from build123d import *

# Parameters (mm, degrees)
F1_DEPTH = 5.8


with BuildPart() as f1:
    # F0 (on Top) → F1 (new body)
    with BuildSketch(Plane.XY):
        Polygon((19.870715, 20.171389), (11.003364, 25.828145), (9.710712, 25.935493), (8.638659, 25.674237), (7.548944, 24.40875), (7.098501, 22.336712), (7.098501, 20.264676), (7.745507, 18.576713), (8.39527, 18.462049), (9.515883, 19.793121), (10.092715, 21.398216), (11.178206, 21.398216), (11.178206, 15.477047), (11.710122, 14.888561), (12.432186, 15.31403), (14.361553, 18.82783), (14.710026, 18.82783), (14.968658, 17.630091), (15.437118, 16.368851), (16.193863, 15.467965), (16.986642, 14.999504), (15.95501, 4.724317), (15.226499, 4.017233), (14.733682, 3.160161), (14.540842, 1.960261), (14.733682, 0.846068), (15.183645, 0), (15.805023, -0.675234), (14.859016, -12.881954), (14.056012, -13.806167), (13.617913, -16.297314), (12.787792, -16.297314), (10.52028, -10.248602), (9.737968, -9.775993), (8.959359, -10.581703), (8.959359, -18.013308), (7.532651, -18.013308), (7.532651, -16.239962), (6.00086, -14.336004), (5.722645, -14.336004), (4.844186, -15.200062), (4.586618, -16.215181), (4.586618, -17.39696), (5.071451, -18.609043), (5.722946, -19.396897), (7.289982, -20.181168), (23.513971, -20.668361), (25.093786, -20.388072), (26.864707, -19.636385), (28.431782, -18.527966), (30.902525, -17.158909), (31.791739, -17.158909), (32.466684, -16.912501), (33.098772, -16.408972), (33.633251, -15.701212), (33.868946, -14.790573), (33.868946, -13.933501), (33.579685, -13.301411), (32.847531, -12.387843), (32.847531, -11.59999), (32.847531, -10.190943), (32.286942, -8.706142), (31.696055, -7.554664), (30.464781, -5.741373), (29.919345, -4.332328), (29.782984, -2.574808), (29.979948, -1.13546), (30.373875, 0.137226), (30.752651, 1.07659), (31.948227, 2.286357), (32.443713, 2.286357), (33.434689, 2.133206), (34.362599, 2.331401), (35.272494, 2.7368), (35.912123, 3.295349), (36.371578, 3.889933), (36.58779, 3.889933), (37.781443, 3.788194), (38.622316, 3.788194), (39.412223, 3.915599), (40.253092, 4.399735), (40.597085, 5.329788), (40.597085, 6.196138), (40.342275, 6.833161), (39.743476, 7.189893), (37.296191, 7.57748), (35.560623, 7.57748), (33.782199, 7.298932), (31.425729, 6.457172), (29.820433, 5.234089), (27.787192, 2.836954), (26.976394, 1.287431), (26.000202, -1.772101), (26.000202, -3.229123), (26.407311, -5.307521), (27.071541, -7.150225), (28.203402, -9.181112), (28.991256, -10.256835), (29.204722, -11.574975), (29.204722, -13.16472), (28.326225, -14.503894), (27.008476, -15.650228), (25.722869, -16.346598), (24.370953, -16.518012), (22.442544, -16.26089), (20.706974, -15.53238), (19.292805, -14.718162), (21.281268, 16.815733), (21.37769, 17.769225), (21.056287, 18.615583), (20.606324, 19.451229), align=None)
    extrude(amount=F1_DEPTH)


solid = f1.part
Design review of the part built by this model. Coordinates are the model's own, in mm. A direction names the side the tool comes from. Round coordinates to 2 decimals unless told otherwise and drop trailing zeros. Write each loop counter-clockwise with the first axis right and the second up, starting at its lowest first coordinate (ties: lowest second). Pieces come first, ordered by that corner, then holes. Notation, with made-up numbers: (49, 46) - (56, 46) arc R29 cw to (56, 84) - close; hole circle Ø3 at (29, -18.5). An arc over 180 degrees is marked (long way). Return JSON: item names as keys, results as strings. Group by question number.
Item 1: The part is to be moulded in two halves that separate along Y. For faces 1 (the face through (34.68, 7.44, 2.86)), 2 (the face through (32.57, -9.46, 2.86)), 3 (the face through (29.65, -17.853, 2.859)), say which applies: pulls with the +Y half, pulls with the -Y half, needs draft (parallel to the pull), parting line crosses it, or undercut.
Item 2: Insertion check: P1, Ø0.7, axis at y = -11.5, z = 4, coming from the +X side; P2, Ø2, axis at x = 27, z = 5, coming from the +Y side; P3, Ø3, axis at x = 20.5, y = 3.5, coming from the +Z side; P4, Ø1.1, axis at x = 8.5, z = 2, coming from the +Y side. Each pin has a flat end and moves straight along its axis. Give the tip position at first contact, or say it passes through.
Item 3: For probe 1 along Y at (x, z) = (23.5, 1); probe 2 along X at (y, z) = (17, 3.05); probe 3 along Y at (x, z) = (33, 0.25), list the stretches that pass through material, from the lowest coordinate up. Write a range as [from, to].
Item 4: We need section B-B on y = 11.5. Write out the cut boundary in (x, z).
Item 5: We need section A-A on x = 18.5. Write out the cut boundary in (y, z).
Item 6: Machinability: for faces 4 (the face through (15.2, 17.01, 2.86)), 5 (the face through (7.099, 21, 3)), 6 (the face through (29.88, -1.87, 2.86)), which of the approach directions +Z, -Z, +X, -X, +Y, -Y give a long, thin tool a straight path to every point of the face, cutting with its end or side? Answer none if there is none.
Model answer:
{
 "1": {"face 1": "pulls with the +Y half", "face 2": "undercut", "face 3": "pulls with the -Y half"},
 "2": {"P1": "stops at x = 32.85", "P2": "stops at y = 3.09", "P3": "stops at z = 5.8", "P4": "stops at y = 25.77"},
 "3": {"probe 1": "y = [-20.67, -16.4]", "probe 2": "x = [11.18, 13.36], [15.2, 21.3]", "probe 3": "y = [-16.49, -12.58], [2.2, 7.02]"},
 "4": {"outline": "(16.64, 0) - (20.95, 0) - (20.95, 5.8) - (16.64, 5.8) - close"},
 "5": {"outline": "(-20.52, 0) - (21.05, 0) - (21.05, 5.8) - (-20.52, 5.8) - close"},
 "6": {"face 4": "+Z, -Z", "face 5": "+Z, -Z, -X, +Y", "face 6": "+Z, -Z, +X"}
}
